The model under review builds one solid part; all positions refer to its coordinate system, in mm. Face numbers are marked on the shaded views. Round coordinates to 2 decimals unless told otherwise and drop trailing zeros. Loops run counter-clockwise (first coordinate to the right, second up) from the corner with the lowest first, then second, coordinate; pieces in that order, holes last. Notation, with made-up numbers: M 6,13.25 L 24,13.25 A32 ccw 24,45.25 Z; hole C 21.5,87.25 d8. An arc over 180 degrees is marked long. Answer as a JSON object with one key per item and string values. Group by question number.
Item 1: Insertion check: P1, Ø2.5, axis at y = 6.5, z = -2.5, coming from the -X side. The pin has a flat end and moves straight along its axis. Give the tip position at first contact, or say it passes through.
Item 2: Consider section C-C (y = 6.35). Give the boundary of the cut face in (x, z) (3 decimals), and give its area (3 significant figures).
Item 3: To check wall thickness, follow line 1 (Y direction, x = -13, z = 0); line 2 (Y direction, x = -10.5, z = 1); line 3 (X direction, y = 8.5, z = 0) (3 decimals). State the ranges of each line that lie inside material, in increasing order.
Item 4: Consider section A-A (z = 0). Give the boundary of the cut face in (x, y) (3 decimals).
Item 5: The part is to be moulded in two halves that separate along Z. For the marked faces 1, 2, 3 and 4, say which applies: +Z half, -Z half, draft (parallel to the pull), parting line (faces both ways), or undercut.
Item 6: Consider section D-D (z = 2.25). Give the boundary of the cut face in (x, y).
Item 7: Consider section B-B (x = -15). Give the boundary of the cut face in (y, z), and give its area (3 significant figures).
```python
from build123d import *

# Parameters (mm, degrees)
SKETCH1_R           = 1
BOSS_EXTRUDE1_DEPTH = 12.7
SKETCH2_R           = 4
CUT_EXTRUDE1_DEPTH  = 10


with BuildPart() as part:
    # Sketch1 → Boss-Extrude1 (new body)
    with BuildSketch(Plane(origin=(0, 0, 0), x_dir=(1, 0, 0), z_dir=(0, 1, 0))):
        with BuildLine():
            Line((-4.055343897, 0.632583633), (-4.075844459, 0.866906139))
            ThreePointArc((-4.075844459, 0.866906139), (-3.83530083, 1.283539926), (-3.361522369, 1.2))
            Line((-3.361522369, 1.2), (-2.761522369, 0.6))
            ThreePointArc((-2.761522369, 0.6), (-2.304491577, 0.509090923), (-2.04560443, 0.89654292))
            Line((-2.04560443, 0.89654292), (-2.04560443, 2.5))
            ThreePointArc((-2.04560443, 2.5), (-3.070730696, 4.974873734), (-5.54560443, 6))
            Line((-5.54560443, 6), (-18, 6))
            Line((-18, 6), (-18, -6))
            Line((-18, -6), (-5.54560443, -6))
            ThreePointArc((-5.54560443, -6), (-3.070730696, -4.974873734), (-2.04560443, -2.5))
            Line((-2.04560443, -2.5), (-2.04560443, -0.89654292))
            ThreePointArc((-2.04560443, -0.89654292), (-2.304491577, -0.509090923), (-2.761522369, -0.6))
            Line((-2.761522369, -0.6), (-3.361522369, -1.2))
            ThreePointArc((-3.361522369, -1.2), (-3.83530083, -1.283539926), (-4.075844459, -0.866906139))
            Line((-4.075844459, -0.866906139), (-4.055343897, -0.632583633))
            ThreePointArc((-4.055343897, -0.632583633), (-4.635, 0), (-4.055343897, 0.632583633))
        make_face()
        with Locations(Location((-8, 0, 0), (0, 0, 270))):
            Circle(SKETCH1_R, mode=Mode.SUBTRACT)
    extrude(amount=BOSS_EXTRUDE1_DEPTH)

    # Sketch2 → Cut-Extrude1 (cut)
    with BuildSketch(Plane.ZY.offset(18)):
        with Locations((0, 6.35)):
            Circle(SKETCH2_R)
    extrude(amount=-CUT_EXTRUDE1_DEPTH, mode=Mode.SUBTRACT)


solid = part.part
```
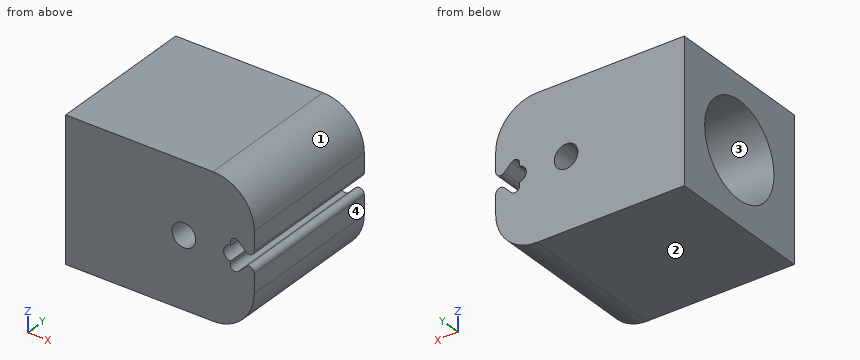
Geometry results:
{
 "1": {"P1": "stops at x = -8"},
 "2": {"outline": "M -18,-6 L -5.546,-6 A3.5 ccw -2.046,-2.5 L -2.046,-0.897 A0.419 ccw -2.762,-0.6 L -3.362,-1.2 A0.419 cw -4.076,-0.867 L -4.055,-0.633 A0.635 cw -4.055,0.633 L -4.076,0.867 A0.419 cw -3.362,1.2 L -2.762,0.6 A0.419 ccw -2.046,0.897 L -2.046,2.5 A3.5 ccw -5.546,6 L -18,6 L -18,4 L -8,4 L -8,1 A1 cw -8,-1 L -8,-4 L -18,-4 Z", "area": "100 mm^2"},
 "3": {"line 1": "y = 0 to 2.35, 10.35 to 12.7", "line 2": "y = 0 to 2.48, 10.22 to 12.7", "line 3": "x = -7 to -4.635"},
 "4": {"outline": "M -18,0 L -9,0 L -9,2.35 L -18,2.35 Z; M -18,10.35 L -9,10.35 L -9,12.7 L -18,12.7 Z; M -7,0 L -4.635,0 L -4.635,12.7 L -7,12.7 Z"},
 "5": {"face 1": "+Z half", "face 2": "-Z half", "face 3": "undercut", "face 4": "draft"},
 "6": {"outline": "M -18,0 L -2.05,0 L -2.05,12.7 L -18,12.7 L -18,9.66 L -8,9.66 L -8,3.04 L -18,3.04 Z"},
 "7": {"outline": "M 0,-6 L 12.7,-6 L 12.7,6 L 0,6 Z; hole C 6.35,0 d8", "area": "102 mm^2"}
}
